Work out the finished part from the listing and answer in its coordinate system (mm). A direction names the side the tool comes from. Coordinates: 2 decimals unless noted, no trailing zeros. Order: outer loops, then holes, each group sorted by start corner. A loop starts at its lowest first (then second) coordinate and runs counter-clockwise, first axis right, second up. Notation, with made-up numbers: (56, 43) -> (72, 43) arc R15 ccw to (72, 67) -> close; hole circle Ø4 at (29, 17). An arc over 180 degrees is marked (long way). Write item = value, one per line. Start each with the question number.
Q1. Flat-ended cylindrical pins translate along their axes: pin 1 (5.5 mm diameter, centred on x = 0, y = 21.92, fed in from +Z); pin 2 (4.5 mm diameter, centred on x = 19, y = 7.5, fed in from -Z). Find the tip coordinate at first contact, or state that the pin passes through.
Q2. The part is cut by section D-D, the plane x = -13. Determine the outline of the cut face in (y, z), plus the area to 3 significant figures.
Q3. The part is cut by section A-A, the plane x = 0. Determine the outline of the cut face in (y, z), plus the area to 3 significant figures.
Q4. The part is cut by section B-B, the plane y = 0. Determine the outline of the cut face in (x, z).
Q5. Straight lines are drawn through the part: L1, parallel to Y at x = 0, z = 7.25; L2, parallel to X at y = -17.5, z = 10.5; L3, parallel to Y at x = -12.5, z = 5. For each, find the intervals that lie inside material, in ascending order. Write a range as from..to.
Q6. Which of the six approach directions +Z, -Z, +X, -X, +Y, -Y give full straight-line access (tool end or side, diameter ignored) to faces 1 (the cylindrical face through (-18.3, 15.1, 3)), 2 (the flat face through (-26.5, -15, 4)), 3 (the cylindrical face through (-0.43, -18.65, 9.04))?
Q7. For a pull along Y with two mould halves and no side action, classify faces 4 (the flat face through (-23.8, -12.4, 4.7)), 5 (the flat face through (-32, 0, 6)), 6 (the flat face through (19, 2.5, 2)) as +Y half, -Y half, draft (parallel to the pull), parting line (faces both ways), or undercut.
Q8. The part is cut by section C-C, the plane z = 10.5. Count the separate pieces of the cut face and the enclosed holes in it, plus the area to 3 significant figures.
```python
from build123d import *

# Parameters (mm, degrees)
SKETCH_W        = 59.5
SKETCH_H        = 66
PAD_DEPTH       = 12
SKETCH001_R     = 3.3
POCKET_DEPTH    = 6
SKETCH002_R     = 3.3
SKETCH002_R_2   = 1.6
POCKET001_DEPTH = 6.001
SKETCH003_R     = 4
POCKET002_DEPTH = 59.501
SKETCH004_R     = 3.3
POCKET003_DEPTH = 5.5
POCKET004_DEPTH = 5.5
SKETCH006_R     = 11.5
POCKET005_DEPTH = 12.001
SKETCH007_W     = 9
SKETCH007_H     = 4
POCKET006_DEPTH = 26


with BuildPart() as part:
    # Sketch → Pad (new body)
    with BuildSketch(Plane.XY):
        with Locations((-2.25, 0)):
            Rectangle(SKETCH_W, SKETCH_H)
    extrude(amount=PAD_DEPTH)

    # Sketch001 (on Face6 of Pad) → Pocket (cut)
    with BuildSketch(Plane.XY.offset(12)):
        with Locations((0, 21.92031)):
            Circle(SKETCH001_R)
        with Locations((-21.92031, 0)):
            Circle(SKETCH001_R)
        with Locations((21.92031, 0)):
            Circle(SKETCH001_R)
        with Locations((0, -21.92031)):
            Circle(SKETCH001_R)
        Polygon((-9.630642, 18.1), (-15, 21.2), (-20.369358, 18.1), (-20.369358, 11.9), (-15, 8.8), (-9.630642, 11.9), align=None)
        Polygon((20.369358, 18.1), (15, 21.2), (9.630642, 18.1), (9.630642, 11.9), (15, 8.8), (20.369358, 11.9), align=None)
        Polygon((-20.369358, -18.1), (-15, -21.2), (-9.630642, -18.1), (-9.630642, -11.9), (-15, -8.8), (-20.369358, -11.9), align=None)
        Polygon((20.369358, -11.9), (15, -8.8), (9.630642, -11.9), (9.630642, -18.1), (15, -21.2), (20.369358, -18.1), align=None)
    extrude(amount=-POCKET_DEPTH, mode=Mode.SUBTRACT)

    # Sketch002 (on Face41 of Pocket) → Pocket001 (cut, through all)
    with BuildSketch(Plane.XY.offset(6)):
        with Locations((-15, 15)):
            Circle(SKETCH002_R)
        with Locations((0, 21.92031)):
            Circle(SKETCH002_R_2)
        with Locations((15, 15)):
            Circle(SKETCH002_R)
        with Locations((-15, -15)):
            Circle(SKETCH002_R)
        with Locations((15, -15)):
            Circle(SKETCH002_R)
        with Locations((0, -21.92031)):
            Circle(SKETCH002_R_2)
        with Locations((21.92031, 0)):
            Circle(SKETCH002_R_2)
        with Locations((-21.92031, 0)):
            Circle(SKETCH002_R_2)
    extrude(amount=-POCKET001_DEPTH, mode=Mode.SUBTRACT)

    # Sketch003 (on Face3 of Pocket001) → Pocket002 (cut, through all)
    with BuildSketch(Plane.YZ.offset(27.5)):
        with Locations((-28, 0)):
            Circle(SKETCH003_R)
        with Locations((28, 0)):
            Circle(SKETCH003_R)
    extrude(amount=-POCKET002_DEPTH, mode=Mode.SUBTRACT)

    # Sketch004 (on Face2 of Pocket002) → Pocket003 (cut)
    with BuildSketch(Plane(origin=(-32, 0, 0), x_dir=(0, -1, 0), z_dir=(-1, 0, 0))):
        with Locations((-15, 0)):
            Circle(SKETCH004_R)
        with Locations((15, 0)):
            Circle(SKETCH004_R)
    extrude(amount=-POCKET003_DEPTH, mode=Mode.SUBTRACT)

    # Sketch005 (on Face42 of Pocket003) → Pocket004 (cut)
    with BuildSketch(Plane(origin=(-26.5, 0, 0), x_dir=(0, -1, 0), z_dir=(-1, 0, 0))):
        Polygon((-9.630642, 3.1), (-15, 6.2), (-20.369358, 3.1), (-20.369358, -3.1), (-15, -6.2), (-9.630642, -3.1), align=None)
        Polygon((9.630642, -3.1), (15, -6.2), (20.369358, -3.1), (20.369358, 3.1), (15, 6.2), (9.630642, 3.1), align=None)
    extrude(amount=-POCKET004_DEPTH, mode=Mode.SUBTRACT)

    # Sketch006 (on Face5 of Pocket004) → Pocket005 (cut, through all)
    with BuildSketch(Plane.XY.offset(12)):
        Circle(SKETCH006_R)
    extrude(amount=-POCKET005_DEPTH, mode=Mode.SUBTRACT)

    # Sketch007 (on Face3 of Pocket005) → Pocket006 (cut)
    with BuildSketch(Plane.YZ.offset(27.5)):
        with Locations((-7, 2)):
            Rectangle(SKETCH007_W, SKETCH007_H)
        with Locations((7, 2)):
            Rectangle(SKETCH007_W, SKETCH007_H)
    extrude(amount=-POCKET006_DEPTH, mode=Mode.SUBTRACT)


solid = part.part
```
Model answer:
q1.pin_1 = 6
q1.pin_2 = 4
q2.outline = (-33, 0) -> (-32, 0) arc R4 cw to (-24, 0) -> (-17.62, 0) -> (-17.62, 6) -> (-20.05, 6) -> (-20.05, 12) -> (-33, 12) -> close; (-12.38, 0) -> (12.38, 0) -> (12.38, 6) -> (9.95, 6) -> (9.95, 12) -> (-9.95, 12) -> (-9.95, 6) -> (-12.38, 6) -> close; (17.62, 0) -> (24, 0) arc R4 cw to (32, 0) -> (33, 0) -> (33, 12) -> (20.05, 12) -> (20.05, 6) -> (17.62, 6) -> close
q2.area = 558 mm2
q3.outline = (-33, 0) -> (-32, 0) arc R4 cw to (-24, 0) -> (-23.52, 0) -> (-23.52, 6) -> (-25.22, 6) -> (-25.22, 12) -> (-33, 12) -> close; (-20.32, 0) -> (-11.5, 0) -> (-11.5, 12) -> (-18.62, 12) -> (-18.62, 6) -> (-20.32, 6) -> close; (11.5, 0) -> (20.32, 0) -> (20.32, 6) -> (18.62, 6) -> (18.62, 12) -> (11.5, 12) -> close; (23.52, 0) -> (24, 0) arc R4 cw to (32, 0) -> (33, 0) -> (33, 12) -> (25.22, 12) -> (25.22, 6) -> (23.52, 6) -> close
q3.area = 348 mm2
q4.outline = (-32, 0) -> (-23.52, 0) -> (-23.52, 6) -> (-25.22, 6) -> (-25.22, 12) -> (-32, 12) -> close; (-20.32, 0) -> (-11.5, 0) -> (-11.5, 12) -> (-18.62, 12) -> (-18.62, 6) -> (-20.32, 6) -> close; (11.5, 0) -> (20.32, 0) -> (20.32, 6) -> (18.62, 6) -> (18.62, 12) -> (11.5, 12) -> close; (23.52, 0) -> (27.5, 0) -> (27.5, 12) -> (25.22, 12) -> (25.22, 6) -> (23.52, 6) -> close
q5.L1 = -33..-25.22, -18.62..-11.5, 11.5..18.62, 25.22..33
q5.L2 = -32..-20.37, -9.63..9.63, 20.37..27.5
q5.L3 = -33..-17.15, -12.85..12.85, 17.15..33
q6.face_1 = +Z, -Z
q6.face_2 = -Z
q6.face_3 = +Z
q7.face_4 = undercut
q7.face_5 = draft
q7.face_6 = undercut
q8.separate_pieces = 1
q8.enclosed_holes = 9
q8.area = 2,980 mm2
